Part model, mm, in its own coordinate system. Face numbers are marked on the shaded views. A direction names the side the tool comes from. Coordinates: 2 decimals unless noted, no trailing zeros. Loops run counter-clockwise (first coordinate to the right, second up) from the corner with the lowest first, then second, coordinate; pieces in that order, holes last. Notation, with made-up numbers: M 28.25,-39.5 L 64.25,-39.5 A14 cw 64.25,-30.5 Z; hole C -38,-8.75 d4. An arc over 180 degrees is marked long. Answer as a JSON object with one key per item and string values. Group by question number.
1. Saw through at D-D on z = 25.5. Write the cut outline in (x, y), then the cut area to 3 significant figures.
2. Saw through at B-B on x = 7.5. Write the cut outline in (y, z), then the cut area to 4 significant figures.
3. Saw through at C-C on y = -0.75. Write the cut outline in (x, z), then the cut area to 3 significant figures.
4. Mould opens along Y. For the marked faces 1, 2 and 3 say: released by +Y, released by -Y, zero draft, split by the parting line, or undercut.
5. Drill centre lines: L1, parallel to Z at x = 9, y = -1.5; L2, parallel to X at y = -4.75, z = 5.5; L3, parallel to Y at x = 13.25, z = 11. Where is each one in solid material? Low to high.
6. Saw through at A-A on z = 6.25. Write the cut outline in (x, y).
7. 3-axis set-ups, long thin cutter, end or side, ignore diameter. For the marked faces 4, 5, 6 and 7: which of +Z, -Z, +X, -X, +Y, -Y reach the whole face in a straight line?
8. Drop flat-ended pins along their axis: pin 1 Ø7.5 at (x, z) = (5, 6) entering from +Y; pin 2 Ø2.5 at (x, y) = (6, -5) entering from +Z; pin 3 Ø3 at (x, z) = (2, 18) entering from -Y. Give the stop position or say it passes through.
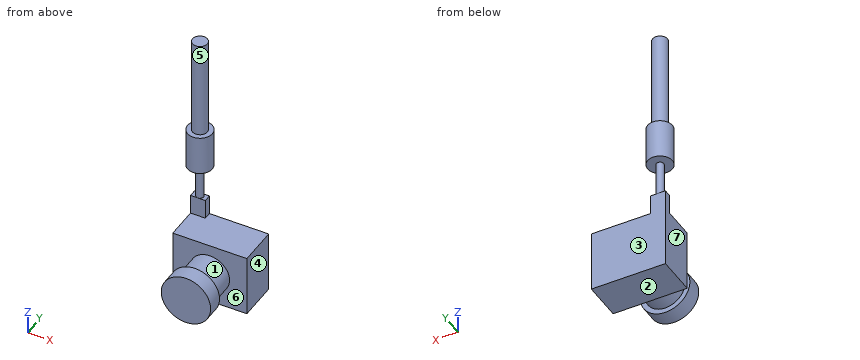
from build123d import *

# Parameters (mm, degrees)
F0_W      = 15
F0_H      = 12.5
F1_DEPTH  = 8
F2_R      = 4
F3_DEPTH  = 5.5
F4_R      = 5
F5_DEPTH  = 3.25
F6_W      = 3
F6_H      = 1.5
F7_DEPTH  = 4
F8_R      = 0.75
F9_DEPTH  = 7
F10_R     = 2.5
F11_DEPTH = 8
F12_R     = 1.5
F13_DEPTH = 20


with BuildPart() as f1:
    # F0 (on Front) → F1 (new body)
    with BuildSketch(Plane.XZ):
        with Locations((7.5, 6.25)):
            Rectangle(F0_W, F0_H)
    extrude(amount=F1_DEPTH)

    # F2 (on face) → F3 (join)
    with BuildSketch(Plane.XZ.offset(8)):
        with Locations((7.5, 6.25)):
            Circle(F2_R)
    extrude(amount=F3_DEPTH)

    # F4 (on face) → F5 (join)
    with BuildSketch(Plane.XZ.offset(13.5)):
        with Locations((7.5, 6.25)):
            Circle(F4_R)
    extrude(amount=F5_DEPTH)

    # F6 (on face) → F7 (join)
    with BuildSketch(Plane.XY.offset(12.5)):
        with Locations((1.5, -0.75)):
            Rectangle(F6_W, F6_H)
    extrude(amount=F7_DEPTH)

    # F8 (on face) → F9 (join)
    with BuildSketch(Plane.XY.offset(16.5)):
        with Locations((1.5, -0.75)):
            Circle(F8_R)
    extrude(amount=F9_DEPTH)

    # F10 (on face) → F11 (join)
    with BuildSketch(Plane.XY.offset(23.5)):
        with Locations((1.5, -0.75)):
            Circle(F10_R)
    extrude(amount=F11_DEPTH)

    # F12 (on face) → F13 (join)
    with BuildSketch(Plane.XY.offset(31.5)):
        with Locations((1.5, -0.75)):
            Circle(F12_R)
    extrude(amount=F13_DEPTH)


solid = f1.part
Outcome:
{
 "1": {"outline": "C 1.5,-0.75 d5", "area": "19.6 mm²"},
 "2": {"outline": "M -16.75,1.25 L -13.5,1.25 L -13.5,2.25 L -8,2.25 L -8,0 L 0,0 L 0,12.5 L -8,12.5 L -8,10.25 L -13.5,10.25 L -13.5,11.25 L -16.75,11.25 Z", "area": "176.5 mm²"},
 "3": {"outline": "M -1,23.5 L 0.75,23.5 L 0.75,16.5 L 0,16.5 L 0,0 L 15,0 L 15,12.5 L 3,12.5 L 3,16.5 L 2.25,16.5 L 2.25,23.5 L 4,23.5 L 4,31.5 L 3,31.5 L 3,51.5 L 0,51.5 L 0,31.5 L -1,31.5 Z", "area": "310 mm²"},
 "4": {"face 1": "undercut", "face 2": "zero draft", "face 3": "released by +Y"},
 "5": {"L1": "z = 0 to 12.5", "L2": "x = 0 to 15", "L3": "y = -8 to 0"},
 "6": {"outline": "M 0,-8 L 3.5,-8 L 3.5,-13.5 L 2.5,-13.5 L 2.5,-16.75 L 12.5,-16.75 L 12.5,-13.5 L 11.5,-13.5 L 11.5,-8 L 15,-8 L 15,0 L 0,0 Z"},
 "7": {"face 4": "+Z, -Z, +X, +Y, -Y", "face 5": "+Z", "face 6": "none", "face 7": "-Z, -X, +Y, -Y"},
 "8": {"pin 1": "stops at y = 0", "pin 2": "stops at z = 12.5", "pin 3": "stops at y = -1.5"}
}
